Check sheet for the modelled part. Datum: model origin and axes. Units: mm. A direction names the side the tool comes from. Give positions to 0.01 mm unless a question says otherwise; leave off trailing zeros. Write each loop counter-clockwise with the first axis right and the second up, starting at its lowest first coordinate (ties: lowest second). Pieces come first, ordered by that corner, then holes. Notation, with made-up numbers: (-16, 33) -> (13, 33) arc R34 cw to (13, 71) -> close; hole circle Ø11 at (0.5, 40.5). An arc over 180 degrees is marked (long way). Return JSON: item names as keys, results as strings.
from build123d import *

# Parameters (mm, degrees)
SKETCH2_R               = 55
BOSS_EXTRUDE1_DEPTH     = 10
SKETCH3_R               = 22.5
BOSS_EXTRUDE2_DEPTH     = 190
SKETCH4_R               = 17.5
CUT_EXTRUDE1_DEPTH      = 1
CUT_EXTRUDE1_DEPTH_BACK = 201
SKETCH14_R              = 37.5
SKETCH14_R_2            = 30.5
CUT_EXTRUDE5_DEPTH      = 1
SKETCH15_R              = 37.5
SKETCH15_R_2            = 30.5
CUT_EXTRUDE6_DEPTH      = 2
SKETCH16_R              = 2.5
CUT_EXTRUDE7_DEPTH      = 4
SKETCH17_R              = 5
CUT_EXTRUDE8_DEPTH      = 2


with BuildPart() as part:
    # Sketch2 → Boss-Extrude1 (new body)
    with BuildSketch(Plane(origin=(0, 0, 0), x_dir=(0, 0, -1), z_dir=(1, 0, 0))):
        Circle(SKETCH2_R)
    extrude(amount=BOSS_EXTRUDE1_DEPTH)

    # Sketch3 → Boss-Extrude2 (add)
    with BuildSketch(Plane(origin=(10, 0, 0), x_dir=(0, 0, -1), z_dir=(1, 0, 0))):
        Circle(SKETCH3_R)
    extrude(amount=BOSS_EXTRUDE2_DEPTH)

    # Sketch4 → Cut-Extrude1 (cut, two sides)
    with BuildSketch(Plane.ZY) as cut_extrude1_sk:
        Circle(SKETCH4_R)
    extrude(amount=CUT_EXTRUDE1_DEPTH, mode=Mode.SUBTRACT)
    extrude(cut_extrude1_sk.sketch, amount=-CUT_EXTRUDE1_DEPTH_BACK, mode=Mode.SUBTRACT)

    # Sketch14 → Cut-Extrude5 (cut)
    with BuildSketch(Plane.ZY):
        Circle(SKETCH14_R)
        Circle(SKETCH14_R_2, mode=Mode.SUBTRACT)
    extrude(amount=-CUT_EXTRUDE5_DEPTH, mode=Mode.SUBTRACT)

    # Sketch15 → Cut-Extrude6 (cut)
    with BuildSketch(Plane(origin=(10, 0, 0), x_dir=(0, 0, -1), z_dir=(1, 0, 0))):
        Circle(SKETCH15_R)
        Circle(SKETCH15_R_2, mode=Mode.SUBTRACT)
    extrude(amount=-CUT_EXTRUDE6_DEPTH, mode=Mode.SUBTRACT)

    # Sketch16 → Cut-Extrude7 (cut)
    with BuildSketch(Plane.ZY):
        with Locations((0, 34)):
            Circle(SKETCH16_R)
        with Locations((0, -34)):
            Circle(SKETCH16_R)
    extrude(amount=-CUT_EXTRUDE7_DEPTH, mode=Mode.SUBTRACT)

    # Sketch17 → Cut-Extrude8 (cut)
    with BuildSketch(Plane.ZY):
        with Locations((0, -34)):
            Circle(SKETCH17_R)
        with Locations((0, 34)):
            Circle(SKETCH17_R)
    extrude(amount=-CUT_EXTRUDE8_DEPTH, mode=Mode.SUBTRACT)


solid = part.part
(1) Depth check by flat-ended pin: pin 1 Ø4 at (y, z) = (-34.5, 1) entering from -X; pin 2 Ø12 at (x, y) = (148.5, -25.5) entering from +Z (3 decimals); pin 3 Ø13 at (y, z) = (-34, 0) entering from +X; pin 4 Ø17 at (y, z) = (-14, -27.5) entering from -X. Enter the tip coordinate at first touch or a pass-through.
Reply:
{"pin 1": "x = 2", "pin 2": "z = 11.225", "pin 3": "x = 10", "pin 4": "x = 0"}
(2) Set-up check for faces 1 (the cylindrical face through (98.6, -10.648, -13.887)), 2 (the cylindrical face through (0.493, 0.623, -30.494)), 3 (the cylindrical face through (9.01, 37.18, 4.88)): record each of +Z, -Z, +X, -X, +Y, -Y from which the full face is reachable in a straight line by a thin tool's end or side.
Reply:
{"face 1": "+X, -X", "face 2": "-X", "face 3": "+X"}
(3) Cross-section at C-C on x = 100. Enter the section's corners in (y, z).
Reply:
{"outline": "circle Ø45 at (0, 0); hole circle Ø35 at (0, 0)"}
(4) Thickness scan on L1, parallel to Y at x = 0.7, z = 0; L2, parallel to Y at x = 2.5, z = 0; L3, parallel to X at y = -42, z = 22. Record the ranges inside material, lowest first.
Reply:
{"L1": "-55 to -39, -29 to -17.5, 17.5 to 29, 39 to 55", "L2": "-55 to -36.5, -31.5 to -17.5, 17.5 to 31.5, 36.5 to 55", "L3": "0 to 10"}
(5) Cross-section at D-D on z = -27. Enter the section's corners in (x, y), then the cut area to 3 significant figures.
Reply:
{"outline": "(0, -47.92) -> (10, -47.92) -> (10, -26.02) -> (8, -26.02) -> (8, -14.19) -> (10, -14.19) -> (10, 14.19) -> (8, 14.19) -> (8, 26.02) -> (10, 26.02) -> (10, 47.92) -> (0, 47.92) -> (0, 26.02) -> (1, 26.02) -> (1, 14.19) -> (0, 14.19) -> (0, -14.19) -> (1, -14.19) -> (1, -26.02) -> (0, -26.02) -> close", "area": "887 mm^2"}
(6) Cross-section at A-A on y = 0. Enter the section's corners in (x, z), then the cut area to 3 significant figures.
Reply:
{"outline": "(0, -55) -> (10, -55) -> (10, -37.5) -> (8, -37.5) -> (8, -30.5) -> (10, -30.5) -> (10, -22.5) -> (200, -22.5) -> (200, -17.5) -> (0, -17.5) -> (0, -30.5) -> (1, -30.5) -> (1, -37.5) -> (0, -37.5) -> close; (0, 17.5) -> (200, 17.5) -> (200, 22.5) -> (10, 22.5) -> (10, 30.5) -> (8, 30.5) -> (8, 37.5) -> (10, 37.5) -> (10, 55) -> (0, 55) -> (0, 37.5) -> (1, 37.5) -> (1, 30.5) -> (0, 30.5) -> close", "area": "2,610 mm^2"}
(7) Cross-section at B-B on z = 7.5. Enter the section's corners in (x, y), then the cut area to 3 significant figures.
Reply:
{"outline": "(0, -54.49) -> (10, -54.49) -> (10, -36.74) -> (8, -36.74) -> (8, -29.56) -> (10, -29.56) -> (10, -21.21) -> (200, -21.21) -> (200, -15.81) -> (0, -15.81) -> (0, -29.56) -> (1, -29.56) -> (1, -36.74) -> (0, -36.74) -> close; (0, 15.81) -> (200, 15.81) -> (200, 21.21) -> (10, 21.21) -> (10, 29.56) -> (8, 29.56) -> (8, 36.74) -> (10, 36.74) -> (10, 54.49) -> (0, 54.49) -> (0, 36.74) -> (1, 36.74) -> (1, 29.56) -> (0, 29.56) -> close", "area": "2,780 mm^2"}
(8) Release check for a two-part mould opening along Y. For faces 4 (the cylindrical face through (103.67, -19.961, -10.382)), 5 (the flat face through (0, -35.9, -11.5)), 6 (the flat face through (8, -30.4, -5.4)) record: pulls with the +Y half, pulls with the -Y half, needs draft (parallel to the pull), parting line crosses it, or undercut.
Reply:
{"face 4": "parting line crosses it", "face 5": "needs draft", "face 6": "undercut"}
